The model under review builds one solid part; all positions refer to its coordinate system, in mm. Face numbers are marked on the shaded views. Give positions to 0.01 mm unless a question says otherwise; leave off trailing zeros. Write each loop counter-clockwise with the first axis right and the second up, starting at its lowest first coordinate (ties: lowest second). Pieces come first, ordered by that corner, then holes. Notation, with made-up numbers: (-4, 10) - (7, 10) arc R8 ccw to (7, 15) - close; hole circle Ø3 at (53, 15). An arc over 180 degrees is marked (long way). Write item = value, one per line.
```python
from build123d import *

# Parameters (mm, degrees)
SKETCH_1_R          = 2.5
EXTRUDE_1_DEPTH     = 2.5
SKETCH_2_OUTSIDE_W  = 52.902
SKETCH_2_OUTSIDE_H  = 39.201
CUT_EXTRUDE_1_DEPTH = 5


with BuildPart() as part:
    # 草圖1 → 填料-伸長1 (new body, symmetric)
    with BuildSketch(Plane.XY):
        with BuildLine():
            Line((28.563543114, 21.665041075), (-2.436456886, 4.366197183))
            ThreePointArc((-2.436456886, 4.366197183), (-4.838955771, -1.258772037), (0, -5))
            Line((0, -5), (20, -5))
            ThreePointArc((20, -5), (22.406799312, -4.382615323), (24.219230218, -2.682926829))
            Line((24.219230218, -2.682926829), (35.219230218, 14.615917063))
            ThreePointArc((35.219230218, 14.615917063), (34.635534008, 20.7314657), (28.563543114, 21.665041075))
        make_face()
        Circle(SKETCH_1_R, mode=Mode.SUBTRACT)
        with Locations((20, 0)):
            Circle(SKETCH_1_R, mode=Mode.SUBTRACT)
        with Locations((31, 17.298843892)):
            Circle(SKETCH_1_R, mode=Mode.SUBTRACT)
    extrude(amount=EXTRUDE_1_DEPTH, both=True)

    # 草圖2 outside → 除料-伸長1 (cut)
    with BuildSketch(Plane.XY.offset(2.5)):
        with Locations((15.5, 8.6495)):
            Rectangle(SKETCH_2_OUTSIDE_W, SKETCH_2_OUTSIDE_H)
        with BuildLine():
            ThreePointArc((1.466809122, 4.780007427), (-4.973314603, -0.515889385), (2.416696414, -4.377165572))
            ThreePointArc((2.416696414, -4.377165572), (10, -2.422785813), (17.583303586, -4.377165572))
            ThreePointArc((17.583303586, -4.377165572), (22.479295807, -4.342014774), (24.997943304, -0.143397121))
            ThreePointArc((24.997943304, -0.143397121), (27.336128289, 7.481863506), (33.249748223, 12.833574255))
            ThreePointArc((33.249748223, 12.833574255), (34.142354704, 21.188009216), (26.161789901, 18.560478956))
            ThreePointArc((26.161789901, 18.560478956), (16.754800429, 6.400785359), (1.466809122, 4.780007427))
        make_face(mode=Mode.SUBTRACT)
    extrude(amount=-CUT_EXTRUDE_1_DEPTH, mode=Mode.SUBTRACT)


solid = part.part
```
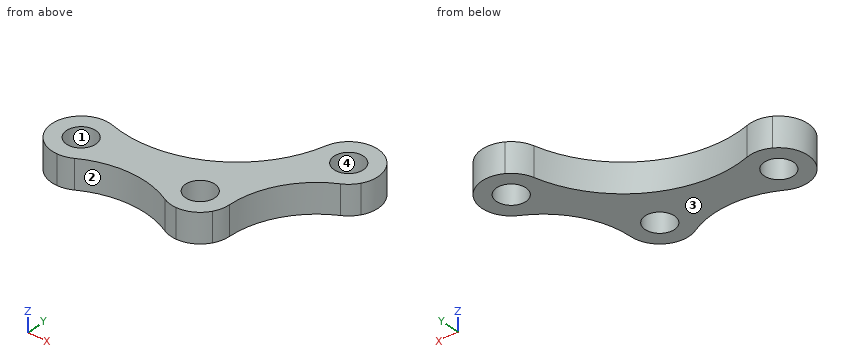
1. Take a section at A-A on x = 18. Give the boundary of the cut face in (y, z), and give its area (3 significant figures).
Findings below:
outline = (-4.58, -2.5) - (-1.5, -2.5) - (-1.5, 2.5) - (-4.58, 2.5) - close; (1.5, -2.5) - (7.16, -2.5) - (7.16, 2.5) - (1.5, 2.5) - close
area = 43.7 mm²
2. Take a section at B-B on z = 1.4. Give the boundary of the cut face in (x, y), and give its area (3 significant figures).
Findings below:
outline = (1.47, 4.78) arc R5 ccw (long way) to (2.42, -4.38) arc R15.69 cw to (17.58, -4.38) arc R5 ccw to (25, -0.14) arc R15.01 cw to (33.25, 12.83) arc R5 ccw (long way) to (26.16, 18.56) arc R19.58 cw to start; hole circle Ø5 at (0, 0); hole circle Ø5 at (20, 0); hole circle Ø5 at (31, 17.3)
area = 343 mm²
3. Draft analysis for pull direction Y (two halves, no side actions). For the marked faces 1, 2, 3 and 4, state which applies: +Y half, -Y half, draft (parallel to the pull), parting line (faces both ways), or undercut.
Findings below:
face_1 = undercut
face_2 = -Y half
face_3 = draft
face_4 = undercut
4. Insertion check: P1, Ø8, axis at x = 16.5, y = 9, coming from the +Z side; P2, Ø3, axis at x = -0.5, z = 0, coming from the +Y side. Each pin has a flat end and moves straight along its axis. Give the tip position at first contact, or say it passes through.
Findings below:
P1 = 2.5
P2 = 5
5. Take a section at C-C on x = 29.5. Give the boundary of the cut face in (y, z).
Findings below:
outline = (10.15, -2.5) - (15.3, -2.5) - (15.3, 2.5) - (10.15, 2.5) - close; (19.3, -2.5) - (22.07, -2.5) - (22.07, 2.5) - (19.3, 2.5) - close
6. For line 1 (Y direction, x = 31, z = -1.2); line 2 (X direction, y = 16.25, z = 0.7); line 3 (X direction, y = 18.75, z = 2.05), list the stretches that pass through material, from the lowest coordinate up. Write a range as from..to.
Findings below:
line_1 = 11.44..14.8, 19.8..22.3
line_2 = 25.4..28.73, 33.27..35.89
line_3 = 26.22..28.96, 33.04..35.78
7. Take a section at D-D on y = 5.5. Give the boundary of the cut face in (x, z).
Findings below:
outline = (14.92, -2.5) - (26.28, -2.5) - (26.28, 2.5) - (14.92, 2.5) - close
